Check sheet for the modelled part. Datum: model origin and axes. Units: mm. A direction names the side the tool comes from. Round coordinates to 2 decimals unless told otherwise and drop trailing zeros. Loops run counter-clockwise (first coordinate to the right, second up) from the corner with the lowest first, then second, coordinate; pieces in that order, holes last. Notation, with made-up numbers: (38.5, -25.75) - (78.5, -25.75) arc R19 ccw to (78.5, -19.75) - close; hole circle Ø3 at (24, -20.5). An arc over 180 degrees is marked (long way). Return JSON: item names as keys, results as strings.
from build123d import *

# Parameters (mm, degrees)
F0_R     = 20
F1_DEPTH = 15
F2_R     = 18
F3_DEPTH = 13
F4_R     = 3.5
F4_R_2   = 1.5
F5_DEPTH = 16
F7_DEPTH = 2


with BuildPart() as f1:
    # F0 (on Top) → F1 (new body)
    with BuildSketch(Plane.XY):
        Circle(F0_R)
    extrude(amount=F1_DEPTH)

    # F2 (on face) → F3 (cut)
    with BuildSketch(Plane.XY.offset(15)):
        Circle(F2_R)
    extrude(amount=-F3_DEPTH, mode=Mode.SUBTRACT)

    # F4 (on face) → F5 (join)
    with BuildSketch(Plane.XY.offset(2)):
        Circle(F4_R)
        Circle(F4_R_2, mode=Mode.SUBTRACT)
    extrude(amount=F5_DEPTH)

    # F6 (on face) → F7 (cut)
    with BuildSketch(Plane(origin=(0, 0, 0), x_dir=(1, 0, 0), z_dir=(0, 0, -1))):
        with BuildLine():
            Line((-15.926695243, 1.5298296101), (-2.9445433001, 2.9445433001))
            Line((-2.9445433001, 2.9445433001), (-1.5298296101, 15.926695243))
            ThreePointArc((-1.5298296101, 15.926695243), (-11.313708499, 11.313708499), (-15.926695243, 1.5298296101))
        make_face()
        with BuildLine():
            Line((-1.5298296101, -15.926695243), (-2.9445433001, -2.9445433001))
            Line((-2.9445433001, -2.9445433001), (-15.926695243, -1.5298296101))
            ThreePointArc((-15.926695243, -1.5298296101), (-11.313708499, -11.313708499), (-1.5298296101, -15.926695243))
        make_face()
        with BuildLine():
            Line((15.926695243, -1.5298296101), (2.9445433001, -2.9445433001))
            Line((2.9445433001, -2.9445433001), (1.5298296101, -15.926695243))
            ThreePointArc((1.5298296101, -15.926695243), (11.313708499, -11.313708499), (15.926695243, -1.5298296101))
        make_face()
        with BuildLine():
            Line((1.5298296101, 15.926695243), (2.9445433001, 2.9445433001))
            Line((2.9445433001, 2.9445433001), (15.926695243, 1.5298296101))
            ThreePointArc((15.926695243, 1.5298296101), (11.313708499, 11.313708499), (1.5298296101, 15.926695243))
        make_face()
    extrude(amount=-F7_DEPTH, mode=Mode.SUBTRACT)


solid = f1.part
Q1. Sectioned sample at A-A (x = -14.5). Enter the section's corners in (y, z).
Answer key:
{"outline": "(-13.77, 0) - (-6.76, 0) - (-6.76, 2) - (-10.67, 2) - (-10.67, 15) - (-13.77, 15) - close; (-1.69, 0) - (1.69, 0) - (1.69, 2) - (-1.69, 2) - close; (6.76, 0) - (13.77, 0) - (13.77, 15) - (10.67, 15) - (10.67, 2) - (6.76, 2) - close"}
Q2. Draft check along X on faces 4 (the face through (-18, 3, 15)), 5 (the face through (2.247, 9.345, 0.986)). Enter one of: released by +X, released by -X, zero draft, split by the parting line, or undercut.
Answer key:
{"face 4": "zero draft", "face 5": "undercut"}
Q3. Scan lines: probe 1 along Y at (x, z) = (0, 6.5); probe 2 along Y at (x, z) = (-2.5, 11); probe 3 along Z at (x, y) = (15, 9). Record each from-to range of solid material in increasing order. Write a range as [from, to].
Answer key:
{"probe 1": "y = [-20, -18], [-3.5, -1.5], [1.5, 3.5], [18, 20]", "probe 2": "y = [-19.84, -17.83], [-2.45, 2.45], [17.83, 19.84]", "probe 3": "z = [0, 2]"}
Q4. Tool access check on faces 1 (the face through (-2.343, 17.847, 8.591)), 2 (the face through (0, -2, 18)), 3 (the face through (-9.526, -2.227, 0.986)). Record the directions out of +Z, -Z, +X, -X, +Y, -Y that give a thin tool (end or side, any length) a straight path to the whole face; none if there is none.
Answer key:
{"face 1": "+Z", "face 2": "+Z, +X, -X, +Y, -Y", "face 3": "+Z, -Z"}
Q5. Sectioned sample at C-C (y = 0). Enter the section's corners in (x, z).
Answer key:
{"outline": "(-20, 0) - (20, 0) - (20, 15) - (18, 15) - (18, 2) - (3.5, 2) - (3.5, 18) - (1.5, 18) - (1.5, 2) - (-1.5, 2) - (-1.5, 18) - (-3.5, 18) - (-3.5, 2) - (-18, 2) - (-18, 15) - (-20, 15) - close"}
Q6. Sectioned sample at D-D (y = -10.5). Enter the section's corners in (x, z).
Answer key:
{"outline": "(-17.02, 0) - (-12.07, 0) - (-12.07, 2) - (-14.62, 2) - (-14.62, 15) - (-17.02, 15) - close; (-2.12, 0) - (2.12, 0) - (2.12, 2) - (-2.12, 2) - close; (12.07, 0) - (17.02, 0) - (17.02, 15) - (14.62, 15) - (14.62, 2) - (12.07, 2) - close"}
Q7. Sectioned sample at B-B (z = 12.75). Enter the section's corners in (x, y), plus the area to 3 significant figures.
Answer key:
{"outline": "circle Ø40 at (0, 0); circle Ø7 at (0, 0); hole circle Ø36 at (0, 0); hole circle Ø3 at (0, 0)", "area": "270 mm²"}
Q8. Depth check by flat-ended pin: P1, Ø1.5, axis at x = 0.5, y = 0, coming from the +Z side; P2, Ø8, axis at x = 7.5, z = 16, coming from the +Y side; P3, Ø4, axis at x = 6, y = 11, coming from the +Z side; P4, Ø6, axis at y = 6.5, z = 13, coming from the -X side. Enter the tip coordinate at first touch or a pass-through.
Answer key:
{"P1": "stops at z = 2", "P2": "stops at y = 19.67", "P3": "passes through", "P4": "stops at x = -19.69"}
